from build123d import *

# Parameters (mm, degrees)
SKETCH1_W           = 100
SKETCH1_H           = 100
BOSS_EXTRUDE1_DEPTH = 8
SKETCH2_W           = 30
SKETCH2_H           = 30
BOSS_EXTRUDE2_DEPTH = 5
SKETCH3_R           = 2
SKETCH3_R_2         = 2.5
CUT_EXTRUDE1_DEPTH  = 19
SKETCH4_R           = 2
SKETCH4_R_2         = 2.5
CUT_EXTRUDE2_DEPTH  = 19
SKETCH5_R           = 2
CUT_EXTRUDE3_DEPTH  = 19
SKETCH6_R           = 2
CUT_EXTRUDE4_DEPTH  = 19


with BuildPart() as part:
    # Sketch1 → Boss-Extrude1 (new body)
    with BuildSketch(Plane(origin=(0, 0, 0), x_dir=(1, 0, 0), z_dir=(0, 1, 0))):
        with Locations((50, 50)):
            Rectangle(SKETCH1_W, SKETCH1_H)
    extrude(amount=BOSS_EXTRUDE1_DEPTH)

    # Sketch2 → Boss-Extrude2 (add)
    with BuildSketch(Plane(origin=(0, 8, 0), x_dir=(1, 0, 0), z_dir=(0, 1, 0))):
        with Locations((50, 50)):
            Rectangle(SKETCH2_W, SKETCH2_H)
    extrude(amount=BOSS_EXTRUDE2_DEPTH)

    # Sketch3 → Cut-Extrude1 (cut)
    with BuildSketch(Plane(origin=(0, 8, 0), x_dir=(1, 0, 0), z_dir=(0, 1, 0))):
        with Locations((10, 90)):
            Circle(SKETCH3_R)
        with Locations((35, 90)):
            Circle(SKETCH3_R)
        with Locations((10, 75)):
            Circle(SKETCH3_R)
        with Locations((35, 75)):
            Circle(SKETCH3_R_2)
    extrude(amount=-CUT_EXTRUDE1_DEPTH, mode=Mode.SUBTRACT)

    # Sketch4 → Cut-Extrude2 (cut)
    with BuildSketch(Plane(origin=(0, 8, 0), x_dir=(1, 0, 0), z_dir=(0, 1, 0))):
        with Locations((90, 85)):
            Circle(SKETCH4_R)
        with Locations((70, 85)):
            Circle(SKETCH4_R_2)
    extrude(amount=-CUT_EXTRUDE2_DEPTH, mode=Mode.SUBTRACT)

    # Sketch5 → Cut-Extrude3 (cut)
    with BuildSketch(Plane(origin=(0, 8, 0), x_dir=(1, 0, 0), z_dir=(0, 1, 0))):
        with Locations((15, 10)):
            Circle(SKETCH5_R)
        with Locations((15, 25)):
            Circle(SKETCH5_R)
        with Locations((15, 40)):
            Circle(SKETCH5_R)
    extrude(amount=-CUT_EXTRUDE3_DEPTH, mode=Mode.SUBTRACT)

    # Sketch6 → Cut-Extrude4 (cut)
    with BuildSketch(Plane(origin=(0, 8, 0), x_dir=(1, 0, 0), z_dir=(0, 1, 0))):
        with Locations((90, 10)):
            Circle(SKETCH6_R)
        with Locations((60, 10)):
            Circle(SKETCH6_R)
        with Locations((75, 18.025911625)):
            Circle(SKETCH6_R)
    extrude(amount=-CUT_EXTRUDE4_DEPTH, mode=Mode.SUBTRACT)


solid = part.part
Part model, mm, in its own coordinate system. A direction names the side the tool comes from. Coordinates: 2 decimals unless noted, no trailing zeros. Loops run counter-clockwise (first coordinate to the right, second up) from the corner with the lowest first, then second, coordinate; pieces in that order, holes last. Notation, with made-up numbers: M 15,-37.5 L 20,-37.5 A20 cw 20,-22.5 Z; hole C 72,67 d6. An arc over 180 degrees is marked long. Use a Markdown table: item, result. Add a question column.
Q1. Cut at B-B (z = -10). Write the cut outline in (x, y), and give its area (3 significant figures).
Q2. Pin check, flat tips, straight feed: P1, Ø5, axis at x = 15, z = -40, coming from the +Y side; P2, Ø1.5, axis at y = 11.5, z = -49, coming from the +X side; P3, Ø4, axis at y = 11, z = -49.5, coming from the -X side. Stop position of each tip, or through.
Q3. Cut at D-D (z = -85). Write the cut outline in (x, y), and give its area (3 significant figures).
Q4. Cut at C-C (z = -40). Write the cut outline in (x, y), and give its area (3 significant figures).
Q5. Mould opens along Z. For faces 1 (the flat face through (50, 10, -65)), 2 (the flat face through (0, 4, -49)), 3 (the cylindrical face through (13.4, 4.1, -23.8)) say: +Z half, -Z half, draft (parallel to the pull), parting line (faces both ways), or undercut.
Q6. Probe L1, parallel to Z at x = 10, y = 5; L2, parallel to Z at x = 15, y = 4; L3, parallel to X at y = 6.25, z = -85. List the from-to ranges inside material, lowest first.
Q7. Which spindle directions (+Z, -Z, +X, -X, +Y, -Y) get a long thin tool onto all of the face, cutting with end or side? Do faces 4 (the flat face through (35, 10, -50)), 5 (the flat face through (65, 10, -50)), 6 (the flat face through (50, 10, -35)). Say none if no direction does.
Q8. Cut at A-A (x = 75). Write the cut outline in (y, z), and give its area (3 significant figures).
Worked out:
| question | item | result |
|---|---|---|
| 1 | outline | M 0,0 L 13,0 L 13,8 L 0,8 Z; M 17,0 L 58,0 L 58,8 L 17,8 Z; M 62,0 L 88,0 L 88,8 L 62,8 Z; M 92,0 L 100,0 L 100,8 L 92,8 Z |
| 1 | area | 704 mm2 |
| 2 | P1 | stops at y = 8 |
| 2 | P2 | stops at x = 65 |
| 2 | P3 | stops at x = 35 |
| 3 | outline | M 0,0 L 67.5,0 L 67.5,8 L 0,8 Z; M 72.5,0 L 88,0 L 88,8 L 72.5,8 Z; M 92,0 L 100,0 L 100,8 L 92,8 Z |
| 3 | area | 728 mm2 |
| 4 | outline | M 0,0 L 13,0 L 13,8 L 0,8 Z; M 17,0 L 100,0 L 100,8 L 65,8 L 65,13 L 35,13 L 35,8 L 17,8 Z |
| 4 | area | 918 mm2 |
| 5 | face 1 | -Z half |
| 5 | face 2 | draft |
| 5 | face 3 | undercut |
| 6 | L1 | z = -100 to -92, -88 to -77, -73 to 0 |
| 6 | L2 | z = -100 to -42, -38 to -27, -23 to -12, -8 to 0 |
| 6 | L3 | x = 0 to 67.5, 72.5 to 88, 92 to 100 |
| 7 | face 4 | +Z, -Z, -X, +Y |
| 7 | face 5 | +Z, -Z, +X, +Y |
| 7 | face 6 | +Z, +X, -X, +Y |
| 8 | outline | M 0,-100 L 8,-100 L 8,-20.03 L 0,-20.03 Z; M 0,-16.03 L 8,-16.03 L 8,0 L 0,0 Z |
| 8 | area | 768 mm2 |
